```python
from build123d import *

# Parameters (mm, degrees)
F0_R     = 2.5
F1_DEPTH = 2
F2_R     = 5


with BuildPart() as f1:
    # F0 (on Front) → F1 (new body)
    with BuildSketch(Plane.XZ):
        Polygon((-25, 7), (0, 7), (0, 50.54388), (0, 70), (-25, 70), align=None)
        with Locations((-15, 15)):
            Circle(F0_R, mode=Mode.SUBTRACT)
        with Locations((-15, 55)):
            Circle(F0_R, mode=Mode.SUBTRACT)
        Polygon((0, 50.54388), (0, 7), (25, 7), (25, 70), (0, 70), align=None)
        with Locations((15, 15)):
            Circle(F0_R, mode=Mode.SUBTRACT)
        with Locations((15, 55)):
            Circle(F0_R, mode=Mode.SUBTRACT)
    extrude(amount=F1_DEPTH)

    # F2
    f2_edges = [f1.edges().sort_by_distance(p)[0] for p in [
        (-25, -1, 70),
        (25, -1, 70),
        (-25, -1, 7),
        (25, -1, 7),
    ]]
    fillet(f2_edges, radius=F2_R)


solid = f1.part
```
Build history of the part. All positions in model axes, mm. Round coordinates to 2 decimals unless told otherwise and drop trailing zeros. Loops run counter-clockwise (first coordinate to the right, second up) from the corner with the lowest first, then second, coordinate; pieces in that order, holes last. Notation, with made-up numbers: M -17.5,82.25 L 24.5,82.25 A20 cw 24.5,98.25 Z; hole C 41,-15 d8. An arc over 180 degrees is marked long. Answer as CSV lines item,"result".
1. Cut at A-A on z = 55. Write the cut outline in (x, y), then the cut area to 3 significant figures.
Resolved:
outline,"M -25,-2 L -17.5,-2 L -17.5,0 L -25,0 Z; M -12.5,-2 L 12.5,-2 L 12.5,0 L -12.5,0 Z; M 17.5,-2 L 25,-2 L 25,0 L 17.5,0 Z"
area,"80.0 mm²"
2. Two-plate mould, pull along Z, no slides. Class faces 1 (the cylindrical face through (-24, -1, 68)), 2 (the cylindrical face through (12.5, -1, 55.1)), 3 (the flat face through (0, 0, 39)): released by +Z, released by -Z, zero draft, split by the parting line, or undercut.
Resolved:
face 1,"released by +Z"
face 2,"undercut"
face 3,"zero draft"
3. Cut at B-B on x = -15. Write the cut outline in (y, z), then the cut area to 3 significant figures.
Resolved:
outline,"M -2,7 L 0,7 L 0,12.5 L -2,12.5 Z; M -2,17.5 L 0,17.5 L 0,52.5 L -2,52.5 Z; M -2,57.5 L 0,57.5 L 0,70 L -2,70 Z"
area,"106 mm²"
4. Flat gauge pin, fed straight in: P1, Ø4, axis at x = -15, z = 15, coming from the -Y side. Where does the tip first touch, or does it go through?
Resolved:
P1,"passes through"
5. Wall check: probe 1 along Z at (x, y) = (-15, -0.75); probe 2 along Z at (x, y) = (13.5, -0.7); probe 3 along X at (y, z) = (-0.05, 13). Give the ranges that are in metal, low to high. Write a range as [from, to].
Resolved:
probe 1,"z = [7, 12.5], [17.5, 52.5], [57.5, 70]"
probe 2,"z = [7, 13], [17, 53], [57, 70]"
probe 3,"x = [-25, -16.5], [-13.5, 13.5], [16.5, 25]"
6. Cut at C-C on y = -1.35. Write the cut outline in (x, z), then the cut area to 3 significant figures.
Resolved:
outline,"M -25,12 A5 ccw -20,7 L 20,7 A5 ccw 25,12 L 25,65 A5 ccw 20,70 L -20,70 A5 ccw -25,65 Z; hole C -15,15 d5; hole C -15,55 d5; hole C 15,15 d5; hole C 15,55 d5"
area,"3,050 mm²"
